Geometry: final body of the model. Coordinates: model frame, mm. A direction names the side the tool comes from. Round coordinates to 2 decimals unless told otherwise and drop trailing zeros. Order: outer loops, then holes, each group sorted by start corner. A loop starts at its lowest first (then second) coordinate and runs counter-clockwise, first axis right, second up. Notation, with made-up numbers: (29, 32) -> (82, 32) arc R29 ccw to (82, 67) -> close; hole circle Ø10 at (50.25, 38.5). An arc over 180 degrees is marked (long way). Put each result on its own line as item: value.
```python
from build123d import *

# Parameters (mm, degrees)
F0_W     = 3
F0_H     = 1000
F1_DEPTH = 2400
F3_DEPTH = 25


with BuildPart() as f1:
    # F0 (on Top) → F1 (new body)
    with BuildSketch(Plane.XY):
        Polygon((0, -50), (0, 0), (-50, 0), (-50, -50), (-47, -50), align=None)
        with Locations((-48.5, -550)):
            Rectangle(F0_W, F0_H)
    extrude(amount=F1_DEPTH)

    # F2 (on face) → F3 (cut)
    with BuildSketch(Plane(origin=(-50, 0, 0), x_dir=(0, -1, 0), z_dir=(-1, 0, 0))):
        with BuildLine():
            Line((507.407176, 2131.650352), (152.407176, 2131.650352))
            ThreePointArc((152.407176, 2131.650352), (143.568342, 2127.989187), (139.907176, 2119.150352))
            ThreePointArc((139.907176, 2119.150352), (143.568342, 2110.311518), (152.407176, 2106.650352))
            Line((152.407176, 2106.650352), (507.407176, 2106.650352))
            ThreePointArc((507.407176, 2106.650352), (516.246011, 2110.311518), (519.907176, 2119.150352))
            ThreePointArc((519.907176, 2119.150352), (516.246011, 2127.989187), (507.407176, 2131.650352))
        make_face()
        with BuildLine():
            Line((871.98, 1781.389432), (516.98, 1781.389432))
            ThreePointArc((516.98, 1781.389432), (508.141165, 1777.728267), (504.48, 1768.889432))
            ThreePointArc((504.48, 1768.889432), (508.141165, 1760.050597), (516.98, 1756.389432))
            Line((516.98, 1756.389432), (871.98, 1756.389432))
            ThreePointArc((871.98, 1756.389432), (880.818834, 1760.050597), (884.48, 1768.889432))
            ThreePointArc((884.48, 1768.889432), (880.818834, 1777.728267), (871.98, 1781.389432))
        make_face()
        with BuildLine():
            Line((647.627461, 1520.91279), (472.627461, 1520.91279))
            ThreePointArc((472.627461, 1520.91279), (463.788626, 1517.251625), (460.127461, 1508.41279))
            ThreePointArc((460.127461, 1508.41279), (463.788626, 1499.573956), (472.627461, 1495.91279))
            Line((472.627461, 1495.91279), (647.627461, 1495.91279))
            ThreePointArc((647.627461, 1495.91279), (656.466296, 1499.573956), (660.127461, 1508.41279))
            ThreePointArc((660.127461, 1508.41279), (656.466296, 1517.251625), (647.627461, 1520.91279))
        make_face()
        with BuildLine():
            Line((426.390964, 1134.527946), (251.390964, 1134.527946))
            ThreePointArc((251.390964, 1134.527946), (242.552129, 1130.86678), (238.890964, 1122.027946))
            ThreePointArc((238.890964, 1122.027946), (242.552129, 1113.189111), (251.390964, 1109.527946))
            Line((251.390964, 1109.527946), (426.390964, 1109.527946))
            ThreePointArc((426.390964, 1109.527946), (435.229799, 1113.189111), (438.890964, 1122.027946))
            ThreePointArc((438.890964, 1122.027946), (435.229799, 1130.86678), (426.390964, 1134.527946))
        make_face()
        with BuildLine():
            Line((934.300172, 916.40743), (409.300172, 916.40743))
            ThreePointArc((409.300172, 916.40743), (400.461338, 912.746265), (396.800172, 903.90743))
            ThreePointArc((396.800172, 903.90743), (400.461338, 895.068595), (409.300172, 891.40743))
            Line((409.300172, 891.40743), (934.300172, 891.40743))
            ThreePointArc((934.300172, 891.40743), (943.139007, 895.068595), (946.800172, 903.90743))
            ThreePointArc((946.800172, 903.90743), (943.139007, 912.746265), (934.300172, 916.40743))
        make_face()
        with BuildLine():
            Line((279.938626, 745.02703), (154.938626, 745.02703))
            ThreePointArc((154.938626, 745.02703), (146.099792, 741.365864), (142.438626, 732.52703))
            ThreePointArc((142.438626, 732.52703), (146.099792, 723.688195), (154.938626, 720.02703))
            Line((154.938626, 720.02703), (279.938626, 720.02703))
            ThreePointArc((279.938626, 720.02703), (288.777461, 723.688195), (292.438626, 732.52703))
            ThreePointArc((292.438626, 732.52703), (288.777461, 741.365864), (279.938626, 745.02703))
        make_face()
        with BuildLine():
            Line((840.819943, 1997.661972), (645.819943, 1997.661972))
            ThreePointArc((645.819943, 1997.661972), (636.981108, 1994.000807), (633.319943, 1985.161972))
            ThreePointArc((633.319943, 1985.161972), (636.981108, 1976.323137), (645.819943, 1972.661972))
            Line((645.819943, 1972.661972), (840.819943, 1972.661972))
            ThreePointArc((840.819943, 1972.661972), (849.658778, 1976.323137), (853.319943, 1985.161972))
            ThreePointArc((853.319943, 1985.161972), (849.658778, 1994.000807), (840.819943, 1997.661972))
        make_face()
        with BuildLine():
            Line((521.740067, 1393.084645), (107.383054, 1393.084645))
            ThreePointArc((107.383054, 1393.084645), (98.54422, 1389.42348), (94.883054, 1380.584645))
            Line((94.883054, 1380.584645), (94.883054, 1355.692506))
            Line((94.883054, 1355.692506), (521.740067, 1355.692506))
            ThreePointArc((521.740067, 1355.692506), (530.578902, 1359.353671), (534.240067, 1368.192506))
            Line((534.240067, 1368.192506), (534.240067, 1380.584645))
            ThreePointArc((534.240067, 1380.584645), (530.578902, 1389.42348), (521.740067, 1393.084645))
        make_face()
    extrude(amount=-F3_DEPTH, mode=Mode.SUBTRACT)


solid = f1.part
```
1. Cut plane D-D on y = -740.5. Return loops of the section in (x, z), and give its area (4 significant figures).
Ans:
outline: (-50, 0) -> (-47, 0) -> (-47, 891.41) -> (-50, 891.41) -> close; (-50, 916.41) -> (-47, 916.41) -> (-47, 1756.39) -> (-50, 1756.39) -> close; (-50, 1781.39) -> (-47, 1781.39) -> (-47, 1972.66) -> (-50, 1972.66) -> close; (-50, 1997.66) -> (-47, 1997.66) -> (-47, 2400) -> (-50, 2400) -> close
area: 6,975 mm²
2. Material intervals for probe 1 along Y at (x, z) = (-12, 1026); probe 2 along X at (y, z) = (-983, 666), sorted ascending.
Ans:
probe 1: -50 to 0
probe 2: -50 to -47
3. Contact query for flat-ended pins moving along their axis: P1, Ø8, axis at x = -11.5, z = 535, coming from the +Y side; P2, Ø1.5, axis at y = -740, z = 1393, coming from the +X side; P3, Ø8, axis at x = -26.5, z = 276, coming from the -Y side. Output: stop coordinate, or through.
Ans:
P1: y = 0
P2: x = -47
P3: y = -50
4. Set-up query: faces 1 (the face through (-47.3, -367, 0)), 2 (the face through (-24, -50, 1183)). Return all of +Z, -Z, +X, -X, +Y, -Y with unobstructed straight access to the full face (end or side cutting, diameter ignored); none if empty.
Ans:
face 1: -Z, +X, -X, +Y, -Y
face 2: +Z, -Z, +X, -Y
5. Cut plane C-C on x = -33.5. Return loops of the section in (y, z).
Ans:
outline: (-50, 0) -> (0, 0) -> (0, 2400) -> (-50, 2400) -> close
6. Cut plane B-B on z = 308. Return loops of the section in (x, y), and give its area (3 significant figures).
Ans:
outline: (-50, -1050) -> (-47, -1050) -> (-47, -50) -> (0, -50) -> (0, 0) -> (-50, 0) -> close
area: 5,500 mm²
7. Cut plane A-A on y = -195. Return loops of the section in (x, z).
Ans:
outline: (-50, 0) -> (-47, 0) -> (-47, 720.03) -> (-50, 720.03) -> close; (-50, 745.03) -> (-47, 745.03) -> (-47, 1355.69) -> (-50, 1355.69) -> close; (-50, 1393.08) -> (-47, 1393.08) -> (-47, 2106.65) -> (-50, 2106.65) -> close; (-50, 2131.65) -> (-47, 2131.65) -> (-47, 2400) -> (-50, 2400) -> close
